```python
from build123d import *

# Parameters (mm, degrees)
SKETCH1_W           = 50
SKETCH1_H           = 34
BOSS_EXTRUDE1_DEPTH = 6
SKETCH2_R           = 1.5
CUT_EXTRUDE1_DEPTH  = 7
CUT_EXTRUDE2_START  = -7
SKETCH3_R           = 1.5
CUT_EXTRUDE2_DEPTH  = 7
CHAMFER1_SIZE       = 2
SKETCH4_R           = 15
CUT_EXTRUDE3_DEPTH  = 3
SKETCH5_R           = 8.5
CUT_EXTRUDE4_DEPTH  = 3


with BuildPart() as part:
    # Sketch1 → Boss-Extrude1 (new body)
    with BuildSketch(Plane(origin=(0, 0, 0), x_dir=(1, 0, 0), z_dir=(0, 1, 0))):
        with Locations((25, 17)):
            Rectangle(SKETCH1_W, SKETCH1_H)
    extrude(amount=BOSS_EXTRUDE1_DEPTH)

    # Sketch2 → Cut-Extrude1 (cut)
    with BuildSketch(Plane(origin=(50, 0, 0), x_dir=(0, 0, -1), z_dir=(1, 0, 0))):
        with Locations((3.75, 3)):
            Circle(SKETCH2_R)
        with Locations((30.25, 3)):
            Circle(SKETCH2_R)
    extrude(amount=-CUT_EXTRUDE1_DEPTH, mode=Mode.SUBTRACT)

    # Sketch3 → Cut-Extrude2 (cut)
    with BuildSketch(Plane.ZY.offset(CUT_EXTRUDE2_START)):
        with Locations(Location((-30.25, 3, 0), (0, 0, 180))):
            Circle(SKETCH3_R)
        with Locations(Location((-3.75, 3, 0), (0, 0, 180))):
            Circle(SKETCH3_R)
    extrude(amount=CUT_EXTRUDE2_DEPTH, mode=Mode.SUBTRACT)

    # Chamfer1
    chamfer1_edges = [part.edges().sort_by_distance(p)[0] for p in [
        (25, 6, -34),
        (25, 6, 0),
    ]]
    chamfer(chamfer1_edges, length=CHAMFER1_SIZE)

    # Sketch4 → Cut-Extrude3 (cut)
    with BuildSketch(Plane.XZ):
        with Locations(Location((25, -17, 0), (0, 0, 270))):
            Circle(SKETCH4_R)
    extrude(amount=-CUT_EXTRUDE3_DEPTH, mode=Mode.SUBTRACT)

    # Sketch5 → Cut-Extrude4 (cut)
    with BuildSketch(Plane.XZ.offset(-3)):
        with Locations(Location((25, -17, 0), (0, 0, 270))):
            Circle(SKETCH5_R)
    extrude(amount=-CUT_EXTRUDE4_DEPTH, mode=Mode.SUBTRACT)


solid = part.part
```
Part model, mm, in its own coordinate system. A direction names the side the tool comes from. Give positions to 0.01 mm unless a question says otherwise; leave off trailing zeros. Write each loop counter-clockwise with the first axis right and the second up, starting at its lowest first coordinate (ties: lowest second). Pieces come first, ordered by that corner, then holes. Notation, with made-up numbers: (-12, 10.5) -> (3, 10.5) arc R27 ccw to (3, 42.5) -> close; hole circle Ø5 at (30, 44). An arc over 180 degrees is marked (long way). Put each result on its own line as item: value. Start each with the question number.
Item 1: Pull direction X, two halves, no side cores. Call faces 4 (the face through (16, 1, -5)), 5 (the face through (3.55, 2.93, -28.75)), 6 (the face through (19.828, 4.479, -10.255)), 7 (the face through (7, 3, -4)): pulls with the +X half, pulls with the -X half, needs draft (parallel to the pull), parting line crosses it, or undercut.
Item 2: Cut at B-B (y = 0.5). List the corners of the cut face in (x, z).
Item 3: Which spindle directions (+Z, -Z, +X, -X, +Y, -Y) get a long thin tool onto all of the face, cutting with end or side? Do faces 1 (the face through (18.5, 3, -23.5)), 2 (the face through (3.55, 2.55, -5.18)), 3 (the face through (43, 3, -30)). Say none if no direction does.
Item 4: Cut at D-D (z = -7). List the corners of the cut face in (x, y).
Item 5: Wall check: L1, parallel to Z at x = 2.5, y = 3; L2, parallel to X at y = 4.75, z = -17; L3, parallel to Y at x = 44.5, z = -3.75. Give the ranges that are in metal, low to high. Write a range as [from, to].
Item 6: Cut at A-A (z = -17). List the corners of the cut face in (x, y), then the cut area to 3 significant figures.
Item 7: Cut at C-C (x = 36.5). List the corners of the cut face in (y, z), then the cut area to 3 significant figures.
Item 8: Pin check, flat tips, straight feed: pin 1 Ø1.8 at (y, z) = (3, -30.25) entering from +X; pin 2 Ø9 at (x, z) = (23.5, -9.5) entering from -Y. Stop position of each tip, or through.
Answer list:
1. face 4: undercut
1. face 5: needs draft
1. face 6: undercut
1. face 7: pulls with the -X half
2. outline: (0, -34) -> (50, -34) -> (50, 0) -> (0, 0) -> close; hole circle Ø30 at (25, -17)
3. face 1: -Y
3. face 2: -X
3. face 3: +X
4. outline: (0, 0) -> (13.82, 0) -> (13.82, 3) -> (36.18, 3) -> (36.18, 0) -> (50, 0) -> (50, 6) -> (0, 6) -> close
5. L1: z = [-34, -31.75], [-28.75, -5.25], [-2.25, 0]
5. L2: x = [0, 16.5], [33.5, 50]
5. L3: y = [0, 1.5], [4.5, 6]
6. outline: (0, 0) -> (10, 0) -> (10, 3) -> (16.5, 3) -> (16.5, 6) -> (0, 6) -> close; (33.5, 3) -> (40, 3) -> (40, 0) -> (50, 0) -> (50, 6) -> (33.5, 6) -> close
6. area: 159 mm2
7. outline: (0, -34) -> (4, -34) -> (6, -32) -> (6, -2) -> (4, 0) -> (0, 0) -> (0, -7.37) -> (3, -7.37) -> (3, -26.63) -> (0, -26.63) -> close
7. area: 142 mm2
8. pin 1: stops at x = 43
8. pin 2: stops at y = 3
